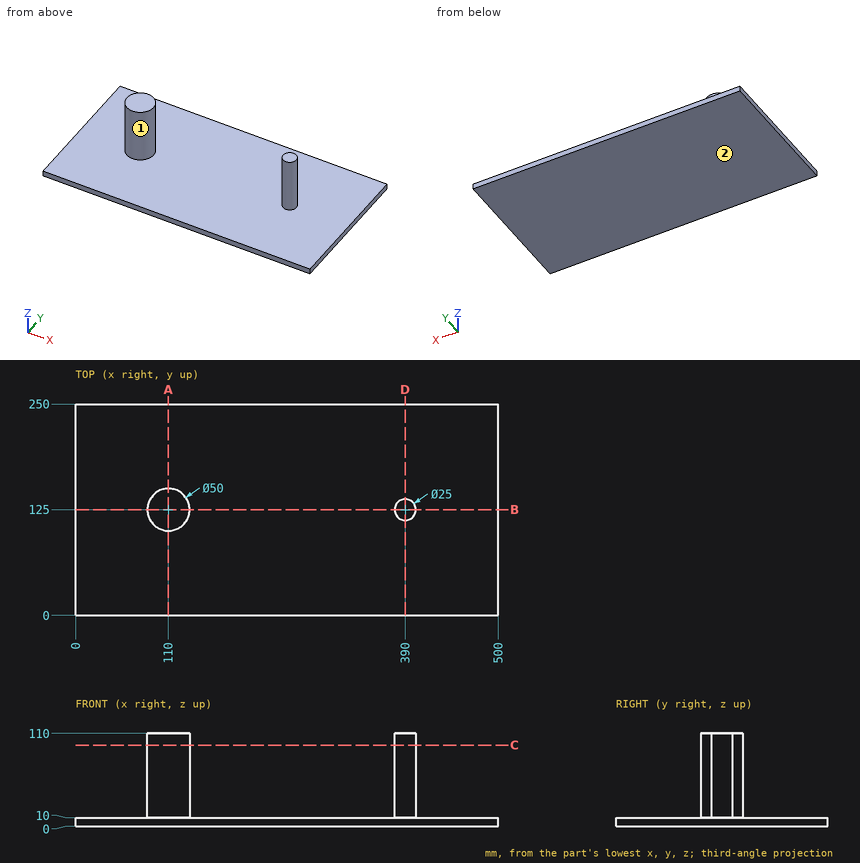
Input: dimensioned drawing with shaded views. Units: mm. Origin: part minimum x, y, z. A direction names the side the tool comes from. Coordinates: 2 decimals unless noted, no trailing zeros. Order: outer loops, then holes, each group sorted by start corner. A loop starts at its lowest first (then second) coordinate and runs counter-clockwise, first axis right, second up. Notation, with made-up numbers: (22, -1.75) - (51, -1.75) arc R31 cw to (51, 26.25) - close; hole circle Ø5 at (-4, 79). An arc over 180 degrees is marked (long way). Return JSON: item names as keys, results as strings. Group by question number.
1. Cut plane D-D (x = 390). Output: boundary loops of the cut face in (y, z).
2. Cut plane A-A (x = 110). Output: boundary loops of the cut face in (y, z).
3. Cut plane B-B (y = 125). Output: boundary loops of the cut face in (x, z), plus the area to 3 significant figures.
4. Cut plane C-C (z = 96). Output: boundary loops of the cut face in (x, y), plus the area to 3 significant figures.
5. Material intervals for line 1 along Z through (x, y) = (183, 95); line 2 along Y through (x, z) = (389, 100); line 3 along X through (y, z) = (130, 101), sorted ascending. Write a range as [from, to].
6. Set-up query: the marked faces 1 and 2. Return all of +Z, -Z, +X, -X, +Y, -Y with unobstructed straight access to the full face (end or side cutting, diameter ignored); none if empty.
7. Pin query (flat end, axial travel): pin 1 (12 mm diameter, centred on x = 106.5, y = 193, fed in from +Z); pin 2 (10 mm diameter, centred on y = 124.5, z = 90.5, fed in from +X); pin 3 (10 mm diameter, centred on x = 386.5, z = 26, fed in from +Y). Return the tip coordinate at first contact, or that it passes through.
Resolved:
{
 "1": {"outline": "(0, 0) - (250, 0) - (250, 10) - (137.5, 10) - (137.5, 110) - (112.5, 110) - (112.5, 10) - (0, 10) - close"},
 "2": {"outline": "(0, 0) - (250, 0) - (250, 10) - (150, 10) - (150, 110) - (100, 110) - (100, 10) - (0, 10) - close"},
 "3": {"outline": "(0, 0) - (500, 0) - (500, 10) - (402.5, 10) - (402.5, 110) - (377.5, 110) - (377.5, 10) - (135, 10) - (135, 110) - (85, 110) - (85, 10) - (0, 10) - close", "area": "12,500 mm²"},
 "4": {"outline": "circle Ø50 at (110, 125); circle Ø25 at (390, 125)", "area": "2,450 mm²"},
 "5": {"line 1": "z = [0, 10]", "line 2": "y = [112.54, 137.46]", "line 3": "x = [85.51, 134.49], [378.54, 401.46]"},
 "6": {"face 1": "+Z", "face 2": "-Z, +X, -X, +Y, -Y"},
 "7": {"pin 1": "stops at z = 10", "pin 2": "stops at x = 402.5", "pin 3": "stops at y = 137.5"}
}
